Read the model definition and answer for the solid it produces. Units are mm, in the model's axes. Give positions to 0.01 mm unless a question says otherwise; leave off trailing zeros. Order: outer loops, then holes, each group sorted by start corner. A loop starts at its lowest first (then second) coordinate and runs counter-clockwise, first axis right, second up. Notation, with made-up numbers: (1, -1.5) -> (9, -1.5) arc R22 ccw to (9, 13.5) -> close; hole circle Ø4 at (69, 56.25). An arc over 180 degrees is marked (long way). One line per item, written item: value. Start each with the question number.
from build123d import *

# Parameters (mm, degrees)
F0_W     = 101.6
F0_H     = 15.875
F0_W_2   = 6.096
F0_H_2   = 152.4
F1_DEPTH = 6.096


with BuildPart() as f1:
    # F0 (on Top) → F1 (new body)
    with BuildSketch(Plane.XY):
        Polygon((63.5, 76.2), (0, 76.2), (-57.404, 76.2), (-57.404, -76.2), (0, -76.2), (63.5, -76.2), align=None)
        with Locations((0, 49.2125)):
            Rectangle(F0_W, F0_H, mode=Mode.SUBTRACT)
        with Locations((-60.452, 0)):
            Rectangle(F0_W_2, F0_H_2)
    extrude(amount=-F1_DEPTH)


solid = f1.part
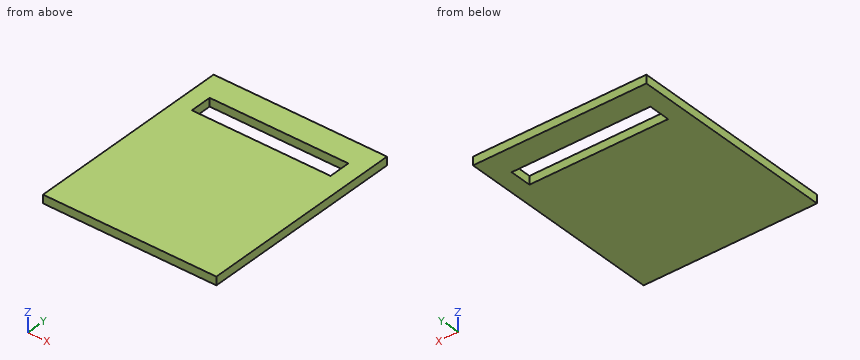
Item 1: Find section A-A on y = 48. Write down the section's boundary in (x, z).
Item 2: Find section B-B on x = -49. Write down the section's boundary in (y, z) (3 decimals), then the cut area to 3 significant figures.
Item 3: Find section C-C on z = -3.25. Write down the section's boundary in (x, y) (3 decimals).
Item 4: Find the intervals of material crossed by line 1 (Y direction, x = -46.5, z = -2.25) (3 decimals); line 2 (X direction, y = 48, z = -1.25), in increasing order. Write a range as from..to.
Checks:
1. outline: (-63.5, -6.1) -> (-50.8, -6.1) -> (-50.8, 0) -> (-63.5, 0) -> close; (50.8, -6.1) -> (63.5, -6.1) -> (63.5, 0) -> (50.8, 0) -> close
2. outline: (-76.2, -6.096) -> (41.275, -6.096) -> (41.275, 0) -> (-76.2, 0) -> close; (57.15, -6.096) -> (76.2, -6.096) -> (76.2, 0) -> (57.15, 0) -> close
2. area: 832 mm2
3. outline: (-63.5, -76.2) -> (63.5, -76.2) -> (63.5, 76.2) -> (-63.5, 76.2) -> close; hole (-50.8, 41.275) -> (50.8, 41.275) -> (50.8, 57.15) -> (-50.8, 57.15) -> close
4. line 1: -76.2..41.275, 57.15..76.2
4. line 2: -63.5..-50.8, 50.8..63.5
